Geometry: final body of the model. Coordinates: model frame, mm. A direction names the side the tool comes from. Give positions to 0.01 mm unless a question says otherwise; leave off trailing zeros. Loops run counter-clockwise (first coordinate to the right, second up) from the corner with the lowest first, then second, coordinate; pieces in that order, holes last.
from build123d import *

# Parameters (mm, degrees)
CROQUIS1_R              = 3.75
CROQUIS1_R_2            = 2.5
SALIENTE_EXTRUIR1_DEPTH = 22.5


with BuildPart() as part:
    # Croquis1 → Saliente-Extruir1 (new body)
    with BuildSketch(Plane.XY):
        with Locations((0.957931978, 153.5)):
            Circle(CROQUIS1_R)
        with Locations((0.957931978, 153.5)):
            Circle(CROQUIS1_R_2, mode=Mode.SUBTRACT)
        with BuildLine():
            ThreePointArc((2, 149.897695982), (1.001580793, 149.750254038), (0, 149.874415037))
            Line((0, 149.874415037), (0, 0))
            Line((0, 0), (2, 7.5))
            Line((2, 7.5), (2, 149.897695982))
        make_face()
    extrude(amount=SALIENTE_EXTRUIR1_DEPTH)


solid = part.part
Item 1: Section query B-B on z = 5. Return loops of the section in (x, y).
Values follow:
outline: (0, 0) - (2, 7.5) - (2, 149.9) arc R3.75 ccw (long way) to (0, 149.87) - close; hole circle Ø5 at (0.96, 153.5)
Item 2: Set-up query: faces 1 (the face through (1, 85, 22.5)), 2 (the face through (0, 76, 11)). Return all of +Z, -Z, +X, -X, +Y, -Y with unobstructed straight access to the full face (end or side cutting, diameter ignored); none if empty.
Values follow:
face 1: +Z, +X, -X, +Y, -Y
face 2: +Z, -Z, -X, -Y
Item 3: Pin query (flat end, axial travel): pin 1 (1.5 mm diameter, centred on y = 71.5, z = 3, fed in from +X); pin 2 (7 mm diameter, centred on y = 107, z = 12, fed in from -X). Return the tip coordinate at first contact, or that it passes through.
Values follow:
pin 1: stops at x = 2
pin 2: stops at x = 0
Item 4: Section query A-A on y = 153.5. Return loops of the section in (x, z).
Values follow:
outline: (-2.79, 0) - (-1.54, 0) - (-1.54, 22.5) - (-2.79, 22.5) - close; (3.46, 0) - (4.71, 0) - (4.71, 22.5) - (3.46, 22.5) - close
Item 5: Ray query, probe 1 along X at (y, z) = (153.5, 12); probe 2 along Y at (x, z) = (3.75, 17.25); probe 3 along X at (y, z) = (92.5, 14.75). Return the intervals inside material, ascending.
Values follow:
probe 1: x = -2.79 to -1.54, 3.46 to 4.71
probe 2: y = 151 to 156
probe 3: x = 0 to 2
Item 6: Section query C-C on y = 131. Return loops of the section in (x, z), plus the area to 3 significant figures.
Values follow:
outline: (0, 0) - (2, 0) - (2, 22.5) - (0, 22.5) - close
area: 45.0 mm2
Item 7: Draft query along Y for faces 3 (the face through (1, 156, 11)), 4 (the face through (2, 78, 11)), 5 (the face through (1.07, 157.25, 11.09)), 6 (the face through (0.986, 3.698, 11.092)). Return one class per face: +Y half, -Y half, draft (parallel to the pull), parting line (faces both ways), or undercut.
Values follow:
face 3: undercut
face 4: draft
face 5: parting line
face 6: -Y half
